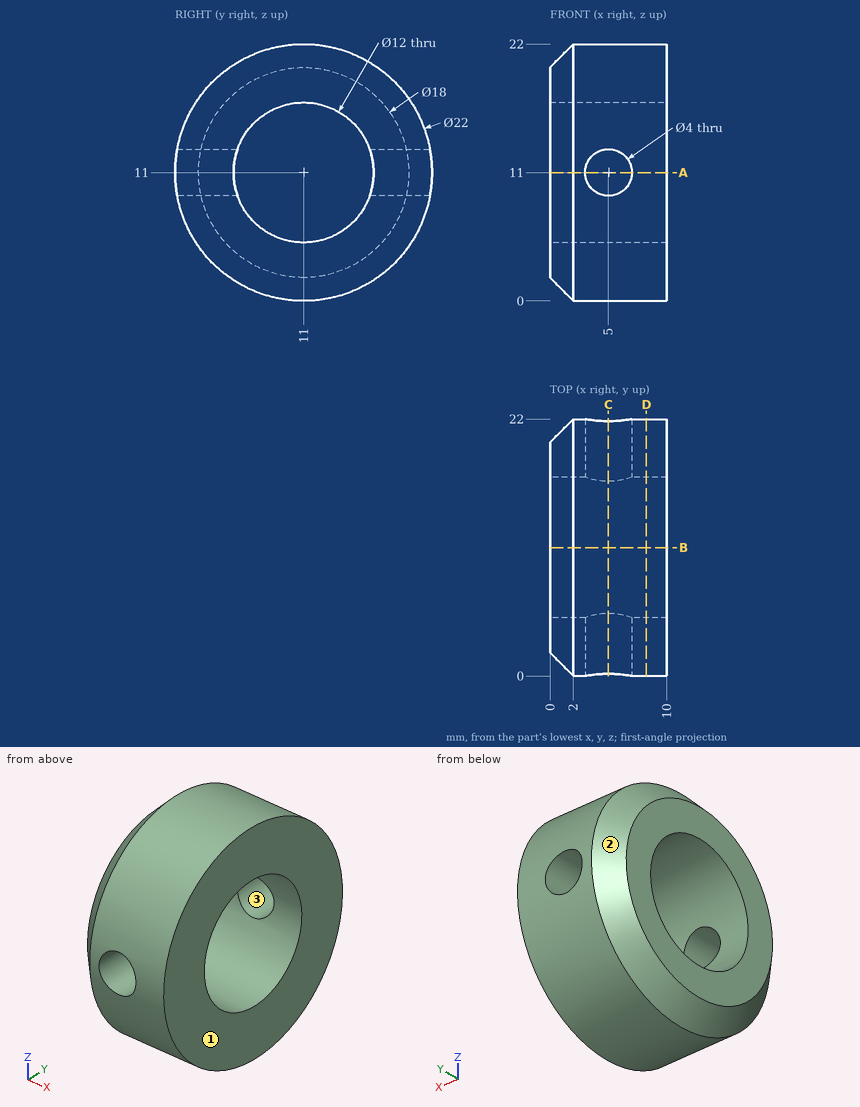
Source: three-view drawing plus pictorial views. Frame: mm from the lowest corner of the part. Round coordinates to 2 decimals unless told otherwise and drop trailing zeros. Loops run counter-clockwise (first coordinate to the right, second up) from the corner with the lowest first, then second, coordinate; pieces in that order, holes last. Notation, with made-up numbers: M 58,72.25 L 107,72.25 A21 ccw 107,82.25 Z; hole C 79.5,-39.75 d4. An arc over 180 degrees is marked long. Put each result on its own line as item: value. Start each with the question number.
(1) Draft query along X for the marked faces 1, 2 and 3. Return one class per face: +X half, -X half, draft (parallel to the pull), parting line (faces both ways), or undercut.
(2) Section query A-A (z = 11). Return loops of the section in (x, y).
(3) Contact query for flat-ended pins moving along their axis: pin 1 Ø1 at (x, y) = (3, 3.5) entering from +Z; pin 2 Ø5 at (x, y) = (3.5, 17.5) entering from +Z; pin 3 Ø3.5 at (x, z) = (5, 11) entering from +Y; pin 4 Ø1 at (x, z) = (8, 6) entering from -Y. Output: stop coordinate, or through.
(4) Section query B-B (y = 11). Return loops of the section in (x, z).
(5) Section query C-C (x = 5). Return loops of the section in (y, z), then the cut area to 3 significant figures.
(6) Section query D-D (x = 8.25). Return loops of the section in (y, z), then the cut area to 3 significant figures.
(7) Material intervals for line 1 along X through (y, z) = (19.05, 11); line 2 along Y through (x, z) = (2.75, 8.5); line 3 along X through (y, z) = (20.75, 10), sorted ascending. Write a range as [from, to].
Findings below:
1. face 1: +X half
1. face 2: -X half
1. face 3: undercut
2. outline: M 0,2 L 2,0 L 3,0 L 3,5 L 0,5 Z; M 0,17 L 3,17 L 3,22 L 2,22 L 0,20 Z; M 7,0 L 10,0 L 10,5 L 7,5 Z; M 7,17 L 10,17 L 10,22 L 7,22 Z
3. pin 1: stops at z = 19.49
3. pin 2: stops at z = 21.25
3. pin 3: passes through
3. pin 4: stops at y = 0.96
4. outline: M 0,2 L 2,0 L 10,0 L 10,5 L 0,5 Z; M 0,17 L 10,17 L 10,22 L 2,22 L 0,20 Z
5. outline: M 0.18,9 A11 ccw 21.82,9 L 16.66,9 A6 cw 5.34,9 Z; M 0.18,13 L 5.34,13 A6 cw 16.66,13 L 21.82,13 A11 ccw Z
5. area: 227 mm2
6. outline: C 11,11 d22; hole C 11,11 d12
6. area: 267 mm2
7. line 1: x = [0, 3], [7, 10]
7. line 2: y = [0.29, 5.55], [16.45, 21.71]
7. line 3: x = [0.8, 3.27], [6.73, 10]
